```python
from build123d import *

# Parameters (mm, degrees)
F0_W     = 38.85378
F0_H     = 41.731834
F1_DEPTH = 40.64
F2_SIZE  = 5.08
F3_SIZE  = 5.08


with BuildPart() as f1:
    # F0 (on Front) → F1 (new body)
    with BuildSketch(Plane.XZ):
        Rectangle(F0_W, F0_H)
    extrude(amount=F1_DEPTH)

    # F2
    f2_edges = [f1.edges().sort_by_distance(p)[0] for p in [
        (-19.42689, -20.32, 20.865917),
        (-19.42689, -20.32, -20.865917),
        (-19.42689, 0, 0),
        (-19.42689, -40.64, 0),
    ]]
    chamfer(f2_edges, length=F2_SIZE)

    # F3
    f3_edges = [f1.edges().sort_by_distance(p)[0] for p in [
        (19.42689, -20.32, -20.865917),
        (19.42689, -20.32, 20.865917),
        (19.42689, 0, 0),
        (19.42689, -40.64, 0),
    ]]
    chamfer(f3_edges, length=F3_SIZE)


solid = f1.part
```
Verification items for the finished model (mm, model axes). Give positions to 0.01 mm unless a question says otherwise; leave off trailing zeros. Order: outer loops, then holes, each group sorted by start corner. A loop starts at its lowest first (then second) coordinate and runs counter-clockwise, first axis right, second up. Notation, with made-up numbers: M 80.5,84 L 127.5,84 A10 cw 127.5,90 Z; hole C 4,-17.75 d1. An arc over 180 degrees is marked long. Return JSON: item names as keys, results as strings. Group by question number.
1) Mould release check, pull along X, two halves, no side actions. Record for faces 1 (the face through (16.922, -2.576, -0.292)), 2 (the face through (0, -20, 20.866)), 3 (the face through (-16.851, -38.136, -0.292)): pulls with the +X half, pulls with the -X half, needs draft (parallel to the pull), parting line crosses it, or undercut.
2) Section check A-A on y = -22.5. Record the cut outline in (x, z).
3) Section check B-B on z = 3.5. Record the cut outline in (x, y).
4) Scan lines: line 1 (X direction, y = -24, z = -16.5); line 2 (Z direction, x = 16, y = -10.5); line 3 (X direction, y = -22, z = -19). Record each from-to range of solid material in increasing order.
Answer block:
{
 "1": {"face 1": "pulls with the +X half", "face 2": "needs draft", "face 3": "pulls with the -X half"},
 "2": {"outline": "M -19.43,-15.79 L -14.35,-20.87 L 14.35,-20.87 L 19.43,-15.79 L 19.43,15.79 L 14.35,20.87 L -14.35,20.87 L -19.43,15.79 Z"},
 "3": {"outline": "M -19.43,-35.56 L -14.35,-40.64 L 14.35,-40.64 L 19.43,-35.56 L 19.43,-5.08 L 14.35,0 L -14.35,0 L -19.43,-5.08 Z"},
 "4": {"line 1": "x = -18.71 to 18.71", "line 2": "z = -19.21 to 19.21", "line 3": "x = -16.21 to 16.21"}
}
